```python
from build123d import *

# Parameters (mm, degrees)
SKETCH1_R           = 1.05
BOSS_EXTRUDE1_DEPTH = 2
SKETCH2_R           = 1
BOSS_EXTRUDE2_DEPTH = 4
SKETCH3_W           = 15.8
SKETCH3_H           = 15.3
BOSS_EXTRUDE3_DEPTH = 2
SKETCH4_W           = 27
SKETCH4_H           = 0.2
CUT_EXTRUDE1_DEPTH  = 79.597789409


with BuildPart() as part:
    # Sketch1 → Boss-Extrude1 (new body)
    with BuildSketch(Plane.XY):
        Polygon((-53.65, -57.3), (-45.65, -57.3), (-45.65, -45.3), (-26.65, -45.3), (-26.65, -30), (-53.65, -30), align=None)
        with Locations((-51.85, -55.5)):
            Circle(SKETCH1_R, mode=Mode.SUBTRACT)
    extrude(amount=BOSS_EXTRUDE1_DEPTH)

    # Sketch2 → Boss-Extrude2 (add)
    with BuildSketch(Plane.XY.offset(2)):
        with Locations((-28.45, -38.7)):
            Circle(SKETCH2_R)
        with Locations((-51.85, -32.1)):
            Circle(SKETCH2_R)
    extrude(amount=-BOSS_EXTRUDE2_DEPTH)

    # Sketch3 → Boss-Extrude3 (add)
    with BuildSketch(Plane.XY.offset(2)):
        with Locations((-34.55, -37.65)):
            Rectangle(SKETCH3_W, SKETCH3_H)
    extrude(amount=BOSS_EXTRUDE3_DEPTH)

    # Sketch4 → Cut-Extrude1 (cut, through all)
    with BuildSketch(Plane(origin=(0, 0, 0), x_dir=(-1, 0, 0), z_dir=(0, 0, -1))):
        with Locations((40.15, -30.1)):
            Rectangle(SKETCH4_W, SKETCH4_H)
    extrude(amount=-CUT_EXTRUDE1_DEPTH, mode=Mode.SUBTRACT)


solid = part.part
```
Geometry check sheet. Reference: the model listing, model coordinates, mm. A direction names the side the tool comes from. Coordinates: 2 decimals unless noted, no trailing zeros. Order: outer loops, then holes, each group sorted by start corner. A loop starts at its lowest first (then second) coordinate and runs counter-clockwise, first axis right, second up.
Item 1: Mould release check, pull along X, two halves, no side actions. Record for faces 1 (the flat face through (-26.65, -38, 2)), 2 (the cylindrical face through (-52.078, -56.525, 0.986)), 3 (the flat face through (-53.65, -44, 1)), 4 (the flat face through (-43, -41, 0)): released by +X, released by -X, zero draft, split by the parting line, or undercut.
Item 2: Depth check by flat-ended pin: pin 1 (3.5 mm diameter, centred on x = -51.85, y = -55.5, fed in from -Z); pin 2 (2 mm diameter, centred on y = -34.5, z = 3.5, fed in from -X); pin 3 (1.5 mm diameter, centred on y = -39.5, z = -1, fed in from +X). Enter the tip coordinate at first touch or a pass-through.
Item 3: Section check C-C (y = -32.1). Enter the section's corners in (x, z), plus the area to 3 significant figures.
Item 4: Section check A-A (y = -55.5). Enter the section's corners in (x, z), plus the area to 3 significant figures.
Item 5: Scan lines: line 1 along Y through (x, z) = (-51.85, 1.25); line 2 along Z through (x, y) = (-37.5, -39.5); line 3 along Z through (x, y) = (-44, -31.75). Record each from-to range of solid material in increasing order.
Item 6: Tool access check on faces 5 (the flat face through (-28, -39, -2)), 6 (the flat face through (-50, -57.3, 1)), 7 (the flat face through (-42.45, -38, 3)), 8 (the flat face through (-36, -45.3, 2)), 9 (the cylindrical face through (-52.587, -31.424, -0.986)). Record the directions out of +Z, -Z, +X, -X, +Y, -Y that give a thin tool (end or side, any length) a straight path to the whole face; none if there is none.
Item 7: Section check B-B (x = -51.85). Enter the section's corners in (y, z), plus the area to 3 significant figures.
Item 8: Section check D-D (x = -28.45). Enter the section's corners in (y, z).
Check sheet entries:
1. face 1: released by +X
1. face 2: undercut
1. face 3: released by -X
1. face 4: zero draft
2. pin 1: stops at z = 0
2. pin 2: stops at x = -42.45
2. pin 3: stops at x = -27.45
3. outline: (-53.65, 0) - (-52.85, 0) - (-52.85, -2) - (-50.85, -2) - (-50.85, 0) - (-26.65, 0) - (-26.65, 4) - (-42.45, 4) - (-42.45, 2) - (-53.65, 2) - close
3. area: 89.6 mm2
4. outline: (-53.65, 0) - (-52.9, 0) - (-52.9, 2) - (-53.65, 2) - close; (-50.8, 0) - (-45.65, 0) - (-45.65, 2) - (-50.8, 2) - close
4. area: 11.8 mm2
5. line 1: y = -57.3 to -56.55, -54.45 to -30.2
5. line 2: z = 0 to 4
5. line 3: z = 0 to 2
6. face 5: -Z, +X, -X, +Y, -Y
6. face 6: +Z, -Z, +X, -X, -Y
6. face 7: +Z, -X, +Y, -Y
6. face 8: +Z, -Z, +X, -Y
6. face 9: -Z
7. outline: (-57.3, 0) - (-56.55, 0) - (-56.55, 2) - (-57.3, 2) - close; (-54.45, 0) - (-33.1, 0) - (-33.1, -2) - (-31.1, -2) - (-31.1, 0) - (-30.2, 0) - (-30.2, 2) - (-54.45, 2) - close
7. area: 54.0 mm2
8. outline: (-45.3, 0) - (-39.7, 0) - (-39.7, -2) - (-37.7, -2) - (-37.7, 0) - (-30.2, 0) - (-30.2, 4) - (-45.3, 4) - close
